Can you work these out from the model? Positions are in its coordinate system, mm. A direction names the side the tool comes from. Coordinates: 2 decimals unless noted, no trailing zeros. Order: outer loops, then holes, each group sorted by start corner. A loop starts at its lowest first (then second) coordinate and runs counter-clockwise, first axis right, second up. Notation, with made-up numbers: (63, 47) -> (86, 47) arc R14 ccw to (86, 64) -> close; hole circle Ø5 at (-15.5, 55). An arc over 180 degrees is marked (long way). Answer in a Markdown table with one row per item.
```python
from build123d import *

# Parameters (mm, degrees)
SKETCH_1_R            = 1.5
SKETCH_1_R_2          = 2.6
EXTRUDE_1_DEPTH       = 2
SKETCH_2_R            = 1.5
SKETCH_2_R_2          = 2.6
EXTRUDE_2_DEPTH       = 2.8
FILLET_1_R            = 0.7
EXTRUDE_START         = -4.5
EXTRUDE_3_DEPTH       = 7
EXTRUDE_START_2       = 2.5
EXTRUDE_3_2_DEPTH     = 7.413746647
EXTRUDE_START_3       = -4
EXTRUDE_3_3_OUTLINE_R = 1.5
EXTRUDE_3_3_DEPTH     = 4
CHAMFER_1_SIZE        = 0.5


with BuildPart() as part:
    # 草图1 → 凸台-拉伸1 (new body)
    with BuildSketch(Plane.XY):
        with BuildLine():
            Line((4.5, 19.3), (4.5, 28.329670691))
            ThreePointArc((4.5, 28.329670691), (0, 34.8), (-4.5, 28.329670691))
            Line((-4.5, 28.329670691), (-4.5, 1.670329309))
            ThreePointArc((-4.5, 1.670329309), (-3.39411255, -3.39411255), (1.670329309, -4.5))
            Line((1.670329309, -4.5), (17.329670691, -4.5))
            ThreePointArc((17.329670691, -4.5), (23.724404724, -0.848528137), (19, 4.8))
            ThreePointArc((19, 4.8), (8.746951673, 9.046951673), (4.5, 19.3))
        make_face()
        Circle(SKETCH_1_R, mode=Mode.SUBTRACT)
        with Locations((19, 0)):
            Circle(SKETCH_1_R, mode=Mode.SUBTRACT)
        with Locations((0, 30)):
            Circle(SKETCH_1_R_2, mode=Mode.SUBTRACT)
    extrude(amount=EXTRUDE_1_DEPTH)

    # 草图2 → 凸台-拉伸2 (add)
    with BuildSketch(Plane.XY.offset(2)):
        with BuildLine():
            Line((-1.4, 25.408703887), (-1.4, 4.591296113))
            ThreePointArc((-1.4, 4.591296113), (-3.39411255, -3.39411255), (4.591296113, -1.4))
            Line((4.591296113, -1.4), (14.408703887, -1.4))
            ThreePointArc((14.408703887, -1.4), (23.799903071, -0.030504201), (14.426868498, 1.458241497))
            Line((14.426868498, 1.458241497), (4.591296113, 1.4))
            ThreePointArc((4.591296113, 1.4), (3.39411255, 3.39411255), (1.4, 4.591296113))
            Line((1.4, 4.591296113), (1.4, 25.408703887))
            ThreePointArc((1.4, 25.408703887), (0, 34.8), (-1.4, 25.408703887))
        make_face()
        Circle(SKETCH_2_R, mode=Mode.SUBTRACT)
        with Locations((0, 30)):
            Circle(SKETCH_2_R_2, mode=Mode.SUBTRACT)
        with Locations((19, 0)):
            Circle(SKETCH_2_R, mode=Mode.SUBTRACT)
    extrude(amount=EXTRUDE_2_DEPTH)

    # 圆角1
    fillet_1_edges = [part.edges().sort_by_distance(p)[0] for p in [
        (-1.4, 15, 4.8),
        (9.5, -1.4, 4.8),
        (9.509082305, 1.429120748, 4.8),
        (1.4, 15, 4.8),
    ]]
    fillet(fillet_1_edges, radius=FILLET_1_R)

    # 凸台-拉伸3: read off the stored shape, not the designer's step
    # 凸台-拉伸3 outline → 凸台-拉伸3 (add)
    with BuildSketch(Plane.YZ.offset(EXTRUDE_START)):
        Polygon((28.329670691, 0), (8, 0), (8, -2.561025334), align=None)
    extrude(amount=EXTRUDE_3_DEPTH)

    # Extrude 3 2 outline → Extrude 3 2 (add)
    with BuildSketch(Plane.YZ.offset(EXTRUDE_START_2)):
        Polygon((28.329670691, 0), (8, 0), (8, -2.561025334), align=None)
    extrude(amount=EXTRUDE_3_2_DEPTH)

    # Extrude 3 3 outline → Extrude 3 3 (cut)
    # profile 1 of 3: a face of its own
    with BuildSketch(Plane.XY.offset(EXTRUDE_START_3)):
        with BuildLine():
            ThreePointArc((4.5, 19.3), (5.923290291, 13.035044837), (9.913746647, 8))
            Line((9.913746647, 8), (9.913746647, 28.329670691))
            Line((9.913746647, 28.329670691), (4.5, 28.329670691))
            Line((4.5, 28.329670691), (4.5, 19.3))
        make_face()
    # profile 2 of 3: a face of its own
    with BuildSketch(Plane.XY.offset(EXTRUDE_START_3)):
        with BuildLine():
            ThreePointArc((6.976689308, 8), (5.469210572, 9.857132985), (4.246086412, 11.912711334))
            ThreePointArc((4.246086412, 11.912711334), (3.209776536, 12.39709927), (2.5, 11.5))
            Line((2.5, 11.5), (2.5, 8))
            Line((2.5, 8), (-4.5, 8))
            Line((-4.5, 8), (-4.5, 1.670329309))
            ThreePointArc((-4.5, 1.670329309), (-3.39411255, -3.39411255), (1.670329309, -4.5))
            Line((1.670329309, -4.5), (17.329670691, -4.5))
            ThreePointArc((17.329670691, -4.5), (23.724404724, -0.848528137), (19, 4.8))
            ThreePointArc((19, 4.8), (14.183362168, 5.62337761), (9.913746647, 8))
            Line((9.913746647, 8), (6.976689308, 8))
        make_face()
        Circle(EXTRUDE_3_3_OUTLINE_R, mode=Mode.SUBTRACT)
        with Locations((19, 0)):
            Circle(EXTRUDE_3_3_OUTLINE_R, mode=Mode.SUBTRACT)
    # profile 3 of 3: a face of its own
    with BuildSketch(Plane.XY.offset(EXTRUDE_START_3)):
        with BuildLine():
            Line((1.992485884, 28.329670691), (-1.992485884, 28.329670691))
            ThreePointArc((-1.992485884, 28.329670691), (0, 27.4), (1.992485884, 28.329670691))
        make_face()
    extrude(amount=EXTRUDE_3_3_DEPTH, mode=Mode.SUBTRACT)

    # 草图6 → 切除-旋转1 (revolve, cut)
    with BuildSketch(Plane(origin=(0, 0, 0), x_dir=(0, 0, -1), z_dir=(1, 0, 0))):
        with BuildLine():
            Line((-5.3904059, 30), (0.4095941, 30))
            ThreePointArc((0.4095941, 30), (-2.4904059, 32.9), (-5.3904059, 30))
        make_face()
    revolve(axis=Axis((0, 30, 4.8), (0, 0, -1)), mode=Mode.SUBTRACT)

    # 倒角1
    chamfer_1_edges = [part.edges().sort_by_distance(p)[0] for p in [
        (-2.6, 30, 4.8),
    ]]
    chamfer(chamfer_1_edges, length=CHAMFER_1_SIZE)


solid = part.part
```
(1) We'd pull the mould along X, two halves only. Please class faces 1 (the flat face through (9, -4.5, 1)), 2 (the flat face through (-1.4, 15, 3)), 3 (the flat face through (2.5, 10, -1)), 4 (the flat face through (-1, 8, -1)): +X half, -X half, draft (parallel to the pull), parting line (faces both ways), or undercut.
Response values:
| item | result |
|---|---|
| face 1 | undercut |
| face 2 | -X half |
| face 3 | undercut |
| face 4 | draft |
(2) Suppose I cut it at B-B (y = 30). Please give me the cut outline in (x, z), and give its area (3 significant figures).
Response values:
| item | result |
|---|---|
| outline | (-4.8, 0) -> (-2.6, 0) -> (-2.6, 1.21) arc R2.9 cw to (-2.6, 3.77) -> (-2.6, 4.3) -> (-3.1, 4.8) -> (-4.8, 4.8) -> close; (2.6, 0) -> (4.8, 0) -> (4.8, 4.8) -> (3.1, 4.8) -> (2.6, 4.3) -> (2.6, 3.77) arc R2.9 cw to (2.6, 1.21) -> close |
| area | 19.8 mm2 |
(3) Suppose I cut it at A-A (y = 0). Please give me the cut outline in (x, z).
Response values:
| item | result |
|---|---|
| outline | (-4.8, 0) -> (-1.5, 0) -> (-1.5, 4.8) -> (-4.8, 4.8) -> close; (1.5, 0) -> (17.5, 0) -> (17.5, 4.8) -> (1.5, 4.8) -> close; (20.5, 0) -> (23.8, 0) -> (23.8, 4.8) -> (20.5, 4.8) -> close |
(4) I need wall thicknesses on line 1 (Y direction, x = 0, z = 0.75); line 2 (X direction, y = 30, z = 0.3); line 3 (Y direction, x = 19, z = 1.85). Which ranges of each line are inside material? Lowest first, please. Write a range as [from, to].
Response values:
| item | result |
|---|---|
| line 1 | [-4.8, -1.5], [1.5, 27.4], [32.6, 34.8] |
| line 2 | [-4.8, -2.6], [2.6, 4.8] |
| line 3 | [-4.8, -1.5], [1.5, 4.8] |
(5) On a 3-axis mill with a long thin cutter (end or side, diameter ignored), from which of +Z, -Z, +X, -X, +Y, -Y can I reach the whole of each face in a straight line? I mean faces 5 (the cylindrical face through (3.23, 12.4, -1.07)), 6 (the flat face through (9, -3, 2)), 7 (the flat face through (8, 8, -1)), 8 (the flat face through (-4.5, 15, 0)). Say none if no direction works.
Response values:
| item | result |
|---|---|
| face 5 | -Z, -Y |
| face 6 | +Z, -Y |
| face 7 | -Z, +X, -X, -Y |
| face 8 | +Z, -Z, -X |
(6) Will these pins go through, and if not, where does the flat tip stop? pin 1 Ø5 at (x, y) = (15, 3) entering from -Z; pin 2 Ø1 at (x, y) = (5.5, 6.5) entering from +Z; pin 3 Ø1.7 at (y, z) = (13, 2.5) entering from -X.
Response values:
| item | result |
|---|---|
| pin 1 | z = 0 |
| pin 2 | z = 2 |
| pin 3 | x = -4.5 |
(7) Suppose I cut it at D-D (y = 15). Please give me the cut outline in (x, z), and give its area (3 significant figures).
Response values:
| item | result |
|---|---|
| outline | (-4.5, -1.68) -> (5.15, -1.68) -> (5.15, 2) -> (1.4, 2) -> (1.4, 4.1) arc R0.7 ccw to (0.7, 4.8) -> (-0.7, 4.8) arc R0.7 ccw to (-1.4, 4.1) -> (-1.4, 2) -> (-4.5, 2) -> close |
| area | 43.1 mm2 |
(8) Suppose I cut it at C-C (x = 0). Please give me the cut outline in (y, z), and give its area (3 significant figures).
Response values:
| item | result |
|---|---|
| outline | (-4.8, 0) -> (-1.5, 0) -> (-1.5, 4.8) -> (-4.8, 4.8) -> close; (1.5, 0) -> (8, 0) -> (8, -2.56) -> (27.4, -0.12) -> (27.4, 1.21) arc R2.9 cw to (27.4, 3.77) -> (27.4, 4.3) -> (26.9, 4.8) -> (1.5, 4.8) -> close; (32.6, 0) -> (34.8, 0) -> (34.8, 4.8) -> (33.1, 4.8) -> (32.6, 4.3) -> (32.6, 3.77) arc R2.9 cw to (32.6, 1.21) -> close |
| area | 175 mm2 |
